Geometry: final body of the model. Coordinates: model frame, mm. A direction names the side the tool comes from. Give positions to 0.01 mm unless a question says otherwise; leave off trailing zeros. Write each loop counter-clockwise with the first axis right and the second up, starting at its lowest first coordinate (ties: lowest second). Pieces come first, ordered by that corner, then holes. Notation, with made-up numbers: (-39, 5.5) - (-23, 5.5) arc R21 cw to (-23, 26.5) - close; hole circle Ø1 at (-21.75, 0.5). An arc over 180 degrees is marked (long way). Return JSON: item names as keys, results as strings.
from build123d import *

# Parameters (mm, degrees)
SKETCH1_R           = 3.4925
SKETCH1_R_2         = 4.699
BOSS_EXTRUDE1_DEPTH = 2.54
SKETCH2_R           = 6.35
BOSS_EXTRUDE2_DEPTH = 12.7
SKETCH4_R           = 4.699
CUT_EXTRUDE1_DEPTH  = 6.35


with BuildPart() as part:
    # Sketch1 → Boss-Extrude1 (new body)
    with BuildSketch(Plane(origin=(0, 0, 0), x_dir=(0, 0, -1), z_dir=(1, 0, 0))):
        with BuildLine():
            Line((-12.189561356, 304.55616), (-13.205358136, 329.93584))
            ThreePointArc((-13.205358136, 329.93584), (26.39485874, 329.14336), (65.615293749, 323.615007727))
            Line((65.615293749, 323.615007727), (60.567963461, 298.721545594))
            ThreePointArc((60.567963461, 298.721545594), (24.364484991, 303.82464), (-12.189561356, 304.55616))
        make_face()
        with Locations((0, 317.5)):
            Circle(SKETCH1_R, mode=Mode.SUBTRACT)
        with Locations((25.379671865, 316.484)):
            Circle(SKETCH1_R_2, mode=Mode.SUBTRACT)
        with Locations((50.596913831, 313.4425024)):
            Circle(SKETCH1_R, mode=Mode.SUBTRACT)
    extrude(amount=BOSS_EXTRUDE1_DEPTH)

    # Sketch2 → Boss-Extrude2 (add)
    with BuildSketch(Plane.ZY):
        with Locations((-25.379671865, 316.484)):
            Circle(SKETCH2_R)
    extrude(amount=BOSS_EXTRUDE2_DEPTH)

    # Sketch4 → Cut-Extrude1 (cut)
    with BuildSketch(Plane(origin=(0, 0, 0), x_dir=(0, 0, -1), z_dir=(1, 0, 0))):
        with Locations((25.379671865, 316.484)):
            Circle(SKETCH4_R)
    extrude(amount=-CUT_EXTRUDE1_DEPTH, mode=Mode.SUBTRACT)


solid = part.part
Q1. Pin query (flat end, axial travel): P1, Ø3, axis at x = -7, z = -28, coming from the -Y side; P2, Ø1.5, axis at x = -4, y = 310, coming from the -Z side; P3, Ø4.5, axis at y = 315.5, z = -26.5, coming from the +X side. Return the tip coordinate at first contact, or that it passes through.
Answer key:
{"P1": "stops at y = 310.23", "P2": "stops at z = -28.11", "P3": "stops at x = -6.35"}
Q2. Mould query, pull axis Z, two halves, no side actions, for faces 1 (the cylindrical face through (-1.967, 311.897, -24.361)), 2 (the flat face through (1.25, 317.07, 12.69)), 3 (the flat face through (2.54, 311, -27)). Classes: pulls with the +Z half, pulls with the -Z half, needs draft (parallel to the pull), parting line crosses it, or undercut.
Answer key:
{"face 1": "undercut", "face 2": "pulls with the +Z half", "face 3": "needs draft"}
Q3. Material intervals for probe 1 along Y at (x, z) = (0.8, 0); probe 2 along Z at (x, y) = (0.85, 317.5); probe 3 along X at (y, z) = (320, -45), sorted ascending. Write a range as [from, to].
Answer key:
{"probe 1": "y = [304.8, 314.01], [320.99, 330.2]", "probe 2": "z = [-64.38, -29.97], [-20.79, -3.49], [3.49, 12.71]", "probe 3": "x = [0, 2.54]"}
Q4. Section query B-B, the plane y = 325. Return the cut outline in (x, z).
Answer key:
{"outline": "(0, -58.37) - (2.54, -58.37) - (2.54, 13.01) - (0, 13.01) - close"}
Q5. Section query A-A, the plane z = 0. Return the cut outline in (x, y).
Answer key:
{"outline": "(0, 304.8) - (2.54, 304.8) - (2.54, 314.01) - (0, 314.01) - close; (0, 320.99) - (2.54, 320.99) - (2.54, 330.2) - (0, 330.2) - close"}
Q6. Set-up query: faces 4 (the flat face through (-6.35, 317, -25)), 5 (the cylindrical face through (1.252, 329.187, -25.842)), 6 (the cylindrical face through (1.252, 303.783, -24.875)). Return all of +Z, -Z, +X, -X, +Y, -Y with unobstructed straight access to the full face (end or side cutting, diameter ignored); none if empty.
Answer key:
{"face 4": "+X", "face 5": "+X, -X, +Y", "face 6": "+X, -X, -Y"}
Q7. Section query D-D, the plane x = -8. Return the cut outline in (y, z), plus the area to 3 significant figures.
Answer key:
{"outline": "circle Ø12.7 at (316.48, -25.38)", "area": "127 mm^2"}
Q8. Section query C-C, the plane z = -26. Return the cut outline in (x, y), plus the area to 3 significant figures.
Answer key:
{"outline": "(-12.7, 310.16) - (0, 310.16) - (0, 303.69) - (2.54, 303.69) - (2.54, 311.83) - (-6.35, 311.83) - (-6.35, 321.14) - (2.54, 321.14) - (2.54, 329.17) - (0, 329.17) - (0, 322.8) - (-12.7, 322.8) - close", "area": "142 mm^2"}
